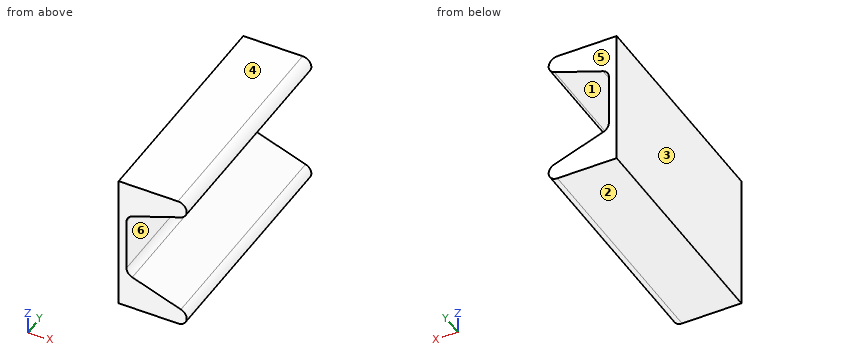
from build123d import *

# Parameters (mm, degrees)
F1_DEPTH = 127


with BuildPart() as f1:
    # F0 (on Front) → F1 (new body)
    with BuildSketch(Plane.XZ):
        with BuildLine():
            Line((0, 38.1), (0, 0))
            Line((0, 0), (32.654806, 0))
            ThreePointArc((32.654806, 0), (37.407898, 3.990299), (34.300957, 9.36257))
            Line((34.300957, 9.36257), (7.514585, 19.082338))
            ThreePointArc((7.514585, 19.082338), (5.196728, 20.858192), (4.318, 23.642784))
            Line((4.318, 23.642784), (4.318, 38.1))
            Line((4.318, 38.1), (4.318, 52.557216))
            ThreePointArc((4.318, 52.557216), (5.196728, 55.341808), (7.514585, 57.117662))
            Line((7.514585, 57.117662), (34.300957, 66.83743))
            ThreePointArc((34.300957, 66.83743), (37.407898, 72.209701), (32.654806, 76.2))
            Line((32.654806, 76.2), (0, 76.2))
            Line((0, 76.2), (0, 38.1))
        make_face()
    extrude(amount=F1_DEPTH)


solid = f1.part
Input: part model. Units: mm. Frame: model coordinates. Face numbers are marked on the shaded views. A direction names the side the tool comes from. Round coordinates to 2 decimals unless told otherwise and drop trailing zeros. Order: outer loops, then holes, each group sorted by start corner. A loop starts at its lowest first (then second) coordinate and runs counter-clockwise, first axis right, second up. Notation, with made-up numbers: (-18.5, 28) - (-4.5, 28) arc R17 ccw to (-4.5, 43) - close; hole circle Ø1 at (37.5, -17). An arc over 180 degrees is marked (long way). Answer as a JSON object with one key per item and string values. Group by question number.
(1) Draft query along Z for the marked faces 1, 2, 3 and 4. Return one class per face: released by +Z, released by -Z, zero draft, split by the parting line, or undercut.
(2) Cut plane C-C (z = 33). Return loops of the section in (x, y).
(3) Reachability of the marked faces 5 and 6 from +Z, -Z, +X, -X, +Y, -Y: full face, straight path, thin tool, end or side. Return the list, or none.
(4) Pin query (flat end, axial travel): P1, Ø14.5, axis at y = -41, z = 42, coming from the +X side. Return the tip coordinate at first contact, or that it passes through.
(5) Material intervals for probe 1 along X at (y, z) = (-81, 50); probe 2 along X at (y, z) = (-39, 5); probe 3 along Z at (x, y) = (5.5, -5.5), sorted ascending. Write a range as from..to.
(6) Cut plane D-D (x = 24). Return loops of the section in (y, z), then the cut area to 3 significant figures.
(7) Cut plane A-A (x = 30). Return loops of the section in (y, z).
(8) Cut plane B-B (y = -32.5). Return loops of the section in (x, z).
Here are the results:
{
 "1": {"face 1": "undercut", "face 2": "released by -Z", "face 3": "zero draft", "face 4": "released by +Z"},
 "2": {"outline": "(0, -127) - (4.32, -127) - (4.32, 0) - (0, 0) - close"},
 "3": {"face 5": "+Z, -Z, +X, -X, +Y", "face 6": "+X, +Y, -Y"},
 "4": {"P1": "stops at x = 4.32"},
 "5": {"probe 1": "x = 0..4.32", "probe 2": "x = 0..37.48", "probe 3": "z = 0..20.47, 55.73..76.2"},
 "6": {"outline": "(-127, 0) - (0, 0) - (0, 13.1) - (-127, 13.1) - close; (-127, 63.1) - (0, 63.1) - (0, 76.2) - (-127, 76.2) - close", "area": "3,330 mm^2"},
 "7": {"outline": "(-127, 0) - (0, 0) - (0, 10.92) - (-127, 10.92) - close; (-127, 65.28) - (0, 65.28) - (0, 76.2) - (-127, 76.2) - close"},
 "8": {"outline": "(0, 0) - (32.65, 0) arc R4.83 ccw to (34.3, 9.36) - (7.51, 19.08) arc R4.85 cw to (4.32, 23.64) - (4.32, 52.56) arc R4.85 cw to (7.51, 57.12) - (34.3, 66.84) arc R4.83 ccw to (32.65, 76.2) - (0, 76.2) - close"}
}
